Verification items for the finished model (mm, model axes). A direction names the side the tool comes from. Round coordinates to 2 decimals unless told otherwise and drop trailing zeros. Write each loop counter-clockwise with the first axis right and the second up, starting at its lowest first coordinate (ties: lowest second). Pieces come first, ordered by that corner, then holes. Notation, with made-up numbers: M -21,78 L 8,78 A14 ccw 8,105 Z; hole C -22,26 d9. An arc over 180 degrees is marked long. Answer in a Markdown table with one row per item. Add a question column.
1. Go/stop test with flat-tipped pins: pin 1 Ø1.5 at (x, y) = (-3, 31) entering from +Z; pin 2 Ø8 at (x, z) = (8, 8) entering from -Y; pin 3 Ø0.6 at (y, z) = (40.5, 22.5) entering from +X. Record where each tip stops, or that it passes through.
2. Material ranges on probe 1 along Z at (x, y) = (-7.75, 37); probe 2 along Z at (x, y) = (2.5, 36.5); probe 3 along Y at (x, z) = (0.25, 17.5), recorded low to high.
3. Sectioned sample at C-C on y = 33.5. Count the separate pieces of the cut face and the enclosed holes in it, plus the area to 3 significant figures.
4. Sectioned sample at B-B on x = -8. Record the cut outline in (y, z), plus the area to 3 significant figures.
5. Set-up check for faces 4 (the cylindrical face through (-11.18, 33.76, 6.54)), 5 (the flat face through (8, 35, 4.75)), 6 (the cylindrical face through (0, 39.7, 30.5)), 7 (the cylindrical face through (-3.52, 35.39, 6.46)): record each of +Z, -Z, +X, -X, +Y, -Y from which the full face is reachable in a straight line by a thin tool's end or side.
6. Sectioned sample at D-D on x = 7.5. Record the cut outline in (y, z), plus the area to 3 significant figures.
7. Draft check along Z on faces 1 (the cylindrical face through (0, 41.7, 16.8)), 2 (the flat face through (0, 36, 0)), 3 (the flat face through (-8, 35, 4.75)). Enter one of: pulls with the +Z half, pulls with the -Z half, needs draft (parallel to the pull), parting line crosses it, or undercut.
8. Sectioned sample at A-A on z = 24.5. Record the cut outline in (x, y), plus the area to 3 significant figures.
```python
from build123d import *

# Parameters (mm, degrees)
EXTRUDE_1_DEPTH          = 27
EXTRUDE_2_DEPTH          = 7
PATTERN_CIRCULAR_1_COUNT = 2
PATTERN_CIRCULAR_1_ANGLE = 7
CUT_EXTRUDE_2_DEPTH      = 1.75
FILLET_1_R               = 1
CHAMFER_1_SIZE           = 1
FILLET_2_R               = 0.5


with BuildPart() as part:
    # Эскиз1 → Бобышка-Вытянуть1 (new body)
    with BuildSketch(Plane.XY):
        with BuildLine():
            Line((10.773634515, 29.600317555), (13.57819969, 37.305797045))
            ThreePointArc((13.57819969, 37.305797045), (8.367171779, 38.808252169), (3, 39.586487594))
            Line((3, 39.586487594), (3, 41.591946336))
            ThreePointArc((3, 41.591946336), (0, 41.7), (-3, 41.591946336))
            Line((-3, 41.591946336), (-3, 39.586487594))
            ThreePointArc((-3, 39.586487594), (-8.367171779, 38.808252169), (-13.57819969, 37.305797045))
            Line((-13.57819969, 37.305797045), (-10.773634515, 29.600317555))
            ThreePointArc((-10.773634515, 29.600317555), (0, 31.5), (10.773634515, 29.600317555))
        make_face()
    extrude(amount=EXTRUDE_1_DEPTH)

    # Эскиз2 → Бобышка-Вытянуть2 (add)
    with BuildSketch(Plane.XY.offset(27)):
        with BuildLine():
            Line((3, 39.586487594), (3, 41.591946336))
            ThreePointArc((3, 41.591946336), (0, 41.7), (-3, 41.591946336))
            Line((-3, 41.591946336), (-3, 39.586487594))
            ThreePointArc((-3, 39.586487594), (0, 39.7), (3, 39.586487594))
        make_face()
    extrude(amount=EXTRUDE_2_DEPTH)

    # Эскиз4 → Вырез-Повернуть1 (revolve, cut)
    with BuildSketch(Plane.XY.offset(6.5)):
        Polygon((13.712080217, 42.895703236), (8.367312695, 23.623094172), (6.680959402, 24.09076133), (12.025726924, 43.363370394), align=None)
    cut_revolve_1 = revolve(axis=Axis((0, 0, 6.5), (0.2672383760782575, 0.9636304532086228, 0)), mode=Mode.SUBTRACT)

    # Круговой массив1: Вырез-Повернуть1 ×2 about axis
    pattern_circular_1_axis = Axis((0, 0, 27), (0, 0, 1))
    for i in range(1, PATTERN_CIRCULAR_1_COUNT):
        add(cut_revolve_1.rotate(pattern_circular_1_axis, i * PATTERN_CIRCULAR_1_ANGLE / (PATTERN_CIRCULAR_1_COUNT - 1)), mode=Mode.SUBTRACT)

    # Эскиз6 → Вырез-Вытянуть2 (cut, symmetric)
    with BuildSketch(Plane.XY.offset(6.5)):
        with BuildLine():
            Line((4.655996451, 31.153999696), (5.868033622, 39.263929775))
            ThreePointArc((5.868033622, 39.263929775), (8.254094125, 38.832459749), (10.60936353, 38.256128992))
            Line((10.60936353, 38.256128992), (8.418008846, 30.354359276))
            ThreePointArc((8.418008846, 30.354359276), (6.549218261, 30.811649423), (4.655996451, 31.153999696))
        make_face()
    cut_extrude_2 = extrude(amount=CUT_EXTRUDE_2_DEPTH, both=True, mode=Mode.SUBTRACT)

    # Зеркальное отражение1: Вырез-Повернуть1, Вырез-Вытянуть2 across plane
    add(cut_revolve_1.mirror(Plane(origin=(0, 0, 0), x_dir=(0, 0, 1), z_dir=(1, 0, 0))), mode=Mode.SUBTRACT)
    add(cut_extrude_2.mirror(Plane(origin=(0, 0, 0), x_dir=(0, 0, 1), z_dir=(1, 0, 0))), mode=Mode.SUBTRACT)

    # Зеркальное отражение1 copy 1 sketch → Зеркальное отражение1 copy 1 (revolve, cut)
    with BuildSketch(Plane(origin=(0, 0, 6.5), x_dir=(-0.992546151641322, 0.12186934340514775, 0), z_dir=(0, 0, 1))):
        Polygon((13.712080217, -42.895703236), (8.367312695, -23.623094172), (6.680959402, -24.09076133), (12.025726924, -43.363370394), align=None)
    revolve(axis=Axis((0, 0, 6.5), (0.147809411129611, -0.9890158633619167, 0)), mode=Mode.SUBTRACT)

    # Скругление1
    fillet_1_edges = [part.edges().sort_by_distance(p)[0] for p in [
        (-3, 39.586487594, 13.5),
        (3, 39.586487594, 13.5),
    ]]
    fillet(fillet_1_edges, radius=FILLET_1_R)

    # Фаска1
    chamfer_1_edges = [part.edges().sort_by_distance(p)[0] for p in [
        (12.175917102, 33.4530573, 0),
        (-12.175917102, 33.4530573, 27),
        (-12.175917102, 33.4530573, 0),
        (12.175917102, 33.4530573, 27),
    ]]
    chamfer(chamfer_1_edges, length=CHAMFER_1_SIZE)

    # Скругление2
    fillet_2_edges = [part.edges().sort_by_distance(p)[0] for p in [
        (-3, 40.589216965, 34),
        (3, 40.589216965, 34),
    ]]
    fillet(fillet_2_edges, radius=FILLET_2_R)


solid = part.part
```
Geometry check:
| question | item | result |
|---|---|---|
| 1 | pin 1 | stops at z = 27 |
| 1 | pin 2 | stops at y = 29.6 |
| 1 | pin 3 | stops at x = 3.05 |
| 2 | probe 1 | z = 0 to 4.75, 8.25 to 27 |
| 2 | probe 2 | z = 0 to 27 |
| 2 | probe 3 | y = 31.5 to 41.7 |
| 3 | separate pieces | 1 |
| 3 | enclosed holes | 2 |
| 3 | area | 607 mm2 |
| 4 | outline | M 30.47,0 L 38.89,0 L 38.89,4.75 L 30.47,4.75 Z; M 30.47,8.25 L 38.89,8.25 L 38.89,27 L 30.47,27 Z |
| 4 | area | 198 mm2 |
| 5 | face 4 | +Y |
| 5 | face 5 | none |
| 5 | face 6 | +Z, -Y |
| 5 | face 7 | -Y |
| 6 | outline | M 30.59,0 L 38.99,0 L 38.99,4.75 L 30.59,4.75 Z; M 30.59,8.25 L 38.99,8.25 L 38.99,27 L 30.59,27 Z |
| 6 | area | 197 mm2 |
| 7 | face 1 | needs draft |
| 7 | face 2 | pulls with the -Z half |
| 7 | face 3 | undercut |
| 8 | outline | M -13.58,37.31 L -10.77,29.6 A31.5 cw 10.77,29.6 L 13.58,37.31 A39.7 ccw 3.9,39.51 A1 cw 3,40.5 L 3,41.59 A41.7 ccw -3,41.59 L -3,40.5 A1 cw -3.9,39.51 A39.7 ccw Z |
| 8 | area | 216 mm2 |
